```python
from build123d import *

# Parameters (mm, degrees)
SKETCH1_R           = 13.4
BOSS_EXTRUDE1_DEPTH = 80
FILLET1_R           = 5
FILLET2_R           = 3
FILLET3_R           = 3
SKETCH2_W           = 97.626120272
SKETCH2_H           = 12
SKETCH2_R           = 1.95
BOSS_EXTRUDE2_DEPTH = 30.8


with BuildPart() as part:
    # Sketch1 → Boss-Extrude1 (new body)
    with BuildSketch(Plane(origin=(0, 0, 0), x_dir=(1, 0, 0), z_dir=(0, 1, 0))):
        Polygon((-17.4, 17.4), (17.4, 17.4), (82.6, 17.4), (82.6, 13.4), (17.4, 13.4), (17.4, -17.4), (-17.4, -17.4), align=None)
        with Locations(Location((0, 0, 0), (0, 0, 270))):
            Circle(SKETCH1_R, mode=Mode.SUBTRACT)
    boss_extrude1 = extrude(amount=BOSS_EXTRUDE1_DEPTH)

    # Mirror3: Boss-Extrude1 across plane
    add(boss_extrude1.mirror(Plane(origin=(82.6, 80, 0), x_dir=(0, 0, 1), z_dir=(1, 0, 0))))

    # Fillet1
    fillet1_edges = [part.edges().sort_by_distance(p)[0] for p in [
        (-17.4, 40, -17.4),
        (182.6, 40, -17.4),
    ]]
    fillet(fillet1_edges, radius=FILLET1_R)

    # Fillet2
    fillet2_edges = [part.edges().sort_by_distance(p)[0] for p in [
        (17.4, 40, 17.4),
        (-17.4, 40, 17.4),
        (147.8, 40, 17.4),
        (182.6, 40, 17.4),
    ]]
    fillet(fillet2_edges, radius=FILLET2_R)

    # Fillet3
    fillet3_edges = [part.edges().sort_by_distance(p)[0] for p in [
        (17.4, 40, -13.4),
        (147.8, 40, -13.4),
    ]]
    fillet(fillet3_edges, radius=FILLET3_R)

    # Sketch2 → Boss-Extrude2 (add)
    # profile 1 of 2: a face of its own
    with BuildSketch(Plane.XY.offset(-13.4)):
        with Locations((92.472437585, 17.5)):
            Rectangle(SKETCH2_W, SKETCH2_H)
        with Locations((52.955461896, 17.190605429)):
            Circle(SKETCH2_R, mode=Mode.SUBTRACT)
        with Locations((134.955461896, 17.190605429)):
            Circle(SKETCH2_R, mode=Mode.SUBTRACT)
    # profile 2 of 2: a face of its own
    with BuildSketch(Plane.XY.offset(-13.4)):
        with Locations((92.472437585, 64.5)):
            Rectangle(SKETCH2_W, SKETCH2_H)
        with Locations((52.955461896, 64.890605429)):
            Circle(SKETCH2_R, mode=Mode.SUBTRACT)
        with Locations((134.955461896, 64.890605429)):
            Circle(SKETCH2_R, mode=Mode.SUBTRACT)
    extrude(amount=BOSS_EXTRUDE2_DEPTH)


solid = part.part
```
Input: part model. Units: mm. Frame: model coordinates. A direction names the side the tool comes from. Coordinates: 2 decimals unless noted, no trailing zeros. Loops run counter-clockwise (first coordinate to the right, second up) from the corner with the lowest first, then second, coordinate; pieces in that order, holes last. Notation, with made-up numbers: M 40.5,36.25 L 81.5,36.25 A22 ccw 81.5,72.25 Z; hole C 46,10.5 d7. An arc over 180 degrees is marked long. Answer in a Markdown table with one row per item.
1. First-contact query: pin 1 (6 mm diameter, centred on x = 134.96, y = 64.89, fed in from +Z); pin 2 (1.9 mm diameter, centred on x = 134.5, y = 65, fed in from +Z); pin 3 (1 mm diameter, centred on x = 133.5, z = 13, fed in from -Y); pin 4 (15.5 mm diameter, centred on x = 82, z = 5, fed in from +Y). Flat tips, straight axial feed; report the tip coordinate or a pass-through.
Response:
| item | result |
|---|---|
| pin 1 | stops at z = 17.4 |
| pin 2 | stops at z = -13.4 |
| pin 3 | stops at y = 11.5 |
| pin 4 | stops at y = 70.5 |
2. Material intervals for line 1 (X direction, y = 21.5, z = 14.5); line 2 (X direction, y = 33, z = 0.5); line 3 (Y direction, x = 130.5, z = -2.5), sorted ascending.
Response:
| item | result |
|---|---|
| line 1 | x = -17.4 to 17.4, 43.66 to 141.29, 147.8 to 182.6 |
| line 2 | x = -17.4 to -13.39, 13.39 to 17.4, 147.8 to 151.81, 178.59 to 182.6 |
| line 3 | y = 11.5 to 23.5, 58.5 to 70.5 |
3. Reachability of faces 1 (the cylindrical face through (51.41, 16, 1.78)), 2 (the flat face through (141.285, 64, 2)), 3 (the flat face through (82, 0, -14)) from +Z, -Z, +X, -X, +Y, -Y: full face, straight path, thin tool, end or side. Return the list, or none.
Response:
| item | result |
|---|---|
| face 1 | +Z |
| face 2 | +Z, +Y, -Y |
| face 3 | +Z, -Z, +X, -X, -Y |
4. Section B-B, the plane z = 11.5. Count the separate pieces of the cut face and the enclosed holes in it, then the cut area to 3 significant figures.
Response:
| item | result |
|---|---|
| separate pieces | 6 |
| enclosed holes | 4 |
| area | 5,660 mm2 |
5. Section C-C, the plane y = 73.5. Output: boundary loops of the cut face in (x, z), then the cut area to 3 significant figures.
Response:
| item | result |
|---|---|
| outline | M -17.4,-12.4 A5 ccw -12.4,-17.4 L 177.6,-17.4 A5 ccw 182.6,-12.4 L 182.6,14.4 A3 ccw 179.6,17.4 L 150.8,17.4 A3 ccw 147.8,14.4 L 147.8,-10.4 A3 cw 144.8,-13.4 L 20.4,-13.4 A3 cw 17.4,-10.4 L 17.4,14.4 A3 ccw 14.4,17.4 L -14.4,17.4 A3 ccw -17.4,14.4 Z; hole C 0,0 d26.8; hole C 165.2,0 d26.8 |
| area | 1,800 mm2 |
6. Draft query along Y for faces 4 (the flat face through (43.659, 64, 2)), 5 (the flat face through (82, 39, -13.4)), 6 (the flat face through (53, 65, -13.4)), 7 (the flat face through (92, 11.5, 2)). Return one class per face: pulls with the +Y half, pulls with the -Y half, needs draft (parallel to the pull), parting line crosses it, or undercut.
Response:
| item | result |
|---|---|
| face 4 | needs draft |
| face 5 | undercut |
| face 6 | undercut |
| face 7 | pulls with the -Y half |
7. Section D-D, the plane x = 72.5. Output: boundary loops of the cut face in (y, z).
Response:
| item | result |
|---|---|
| outline | M 0,-17.4 L 80,-17.4 L 80,-13.4 L 70.5,-13.4 L 70.5,17.4 L 58.5,17.4 L 58.5,-13.4 L 23.5,-13.4 L 23.5,17.4 L 11.5,17.4 L 11.5,-13.4 L 0,-13.4 Z |
8. Section A-A, the plane x = 0. Output: boundary loops of the cut face in (y, z).
Response:
| item | result |
|---|---|
| outline | M 0,-17.4 L 80,-17.4 L 80,-13.4 L 0,-13.4 Z; M 0,13.4 L 80,13.4 L 80,17.4 L 0,17.4 Z |
